Part model, mm, in its own coordinate system. A direction names the side the tool comes from. Give positions to 0.01 mm unless a question says otherwise; leave off trailing zeros. Order: outer loops, then holes, each group sorted by start corner. A loop starts at its lowest first (then second) coordinate and runs counter-clockwise, first axis right, second up. Notation, with made-up numbers: M 56,0.5 L 68,0.5 A22 ccw 68,24.5 Z; hole C -21,78.25 d4. An arc over 180 degrees is marked long. Return JSON: item names as keys, results as strings.
Autodesk Inventor part; units mm, degrees
ref_plane "YZ Plane" through (0, 0, 0) normal (1, 0, 0) x (0, 1, 0)
ref_plane "XZ Plane" through (0, 0, 0) normal (0, 1, 0) x (-1, 0, 0)
ref_plane "XY Plane" through (0, 0, 0) normal (0, 0, 1) x (1, 0, 0)
sketch "Sketch1" plane through (0, 0, 0) normal (0, 1, 0) x (-1, 0, 0)
  line L0 (-20, -20) -> (20, -20)
  line L1 (20, -20) -> (20, 20)
  line L2 (20, 20) -> (-20, 20)
  line L3 (-20, 20) -> (-20, -20)
  line L4 (-20, -20) -> (20, 20) construction
  line L5 (20, -20) -> (-20, 20) construction
  point P0 (0, 0)
  dimension "d2" = 40
  dimension "d3" = 40
extrude "Extrusion1" add sketch "Sketch1" along normal blind 5
sketch "Sketch2" plane through (0, 5, 0) normal (0, 1, 0) x (1, 0, 0)
  line L0 (-20, 20) -> (-20, -20)
  line L1 (-20, -20) -> (20, -20)
  line L2 (20, -20) -> (20, 20)
  line L3 (20, 20) -> (-20, 20)
  line L4 (17, 17) -> (-17, 17)
  line L5 (-17, 17) -> (-17, -17)
  line L6 (-17, -17) -> (17, -17)
  line L7 (17, -17) -> (17, 17)
  line L8 (17, 17) -> (-17, -17) construction
  line L9 (-17, 17) -> (17, -17) construction
  line L10 (15, 15) -> (-15, 15)
  line L11 (-15, 15) -> (-15, -15)
  line L12 (-15, -15) -> (15, -15)
  line L13 (15, -15) -> (15, 15)
  line L14 (15, 15) -> (-15, -15) construction
  line L15 (-15, 15) -> (15, -15) construction
  point P0 (0, 0)
  dimension "d6" = 3
  dimension "d7" = 2
  dimension "d52" = 3
  dimension "d53" = 2
extrude "Extrusion2" add sketch "Sketch2" along normal blind 40 contours L7 L6 L5 L4
fillet "Fillet1" radius 1 1 edges at (20, 2.5, 20)
fillet "Fillet2" radius 1 1 edges at (20, 2.5, -20)
fillet "Fillet3" radius 1 1 edges at (-20, 2.5, 20)
fillet "Fillet4" radius 1 1 edges at (-20, 2.5, -20)
fillet "Fillet5" radius 1 1 edges at (-17, 25, 17)
fillet "Fillet6" radius 1 1 edges at (17, 25, 17)
fillet "Fillet7" radius 1 1 edges at (17, 25, -17)
fillet "Fillet8" radius 1 1 edges at (-17, 25, -17)
sketch "Sketch3" plane through (0, 45, 0) normal (0, 1, 0) x (1, 0, 0)
  arc A0 (-16, 17) -> (-17, 16) centre (-16, 16) ccw
  line L0 (-17, 16) -> (-17, -16)
  arc A1 (-17, -16) -> (-16, -17) centre (-16, -16) ccw
  line L1 (-16, -17) -> (16, -17)
  arc A2 (16, -17) -> (17, -16) centre (16, -16) ccw
  line L2 (17, -16) -> (17, 16)
  arc A3 (17, 16) -> (16, 17) centre (16, 16) ccw
  line L3 (16, 17) -> (-16, 17)
  line L4 (15, 15) -> (15, -15)
  line L5 (15, -15) -> (-15, -15)
  line L6 (-15, -15) -> (-15, 15)
  line L7 (-15, 15) -> (15, 15)
  line L8 (-16.5, -10) -> (-15.5, -10)
  line L9 (-15.5, -10) -> (-15.5, 10)
  line L10 (-15.5, 10) -> (-16.5, 10)
  line L11 (-16.5, 10) -> (-16.5, -10)
  line L12 (-16.5, 10) -> (-15.5, 10)
  line L13 (-15.5, 10) -> (-15.5, -10)
  line L14 (-15.5, -10) -> (-16.5, -10)
  line L15 (-16.5, -10) -> (-16.5, 10)
  line L16 (-10, 16.5) -> (10, 16.5)
  line L17 (10, 16.5) -> (10, 15.5)
  line L18 (10, 15.5) -> (-10, 15.5)
  line L19 (-10, 15.5) -> (-10, 16.5)
  line L20 (10, 16.5) -> (-10, 16.5)
  line L21 (-10, 16.5) -> (-10, 15.5)
  line L22 (-10, 15.5) -> (10, 15.5)
  line L23 (10, 15.5) -> (10, 16.5)
  line L24 (15.5, 10) -> (16.5, 10)
  line L25 (16.5, 10) -> (16.5, -10)
  line L26 (16.5, -10) -> (15.5, -10)
  line L27 (15.5, -10) -> (15.5, 10)
  line L28 (15.5, -10) -> (16.5, -10)
  line L29 (16.5, -10) -> (16.5, 10)
  line L30 (16.5, 10) -> (15.5, 10)
  line L31 (15.5, 10) -> (15.5, -10)
  line L32 (10, -15.5) -> (-10, -15.5)
  line L33 (-10, -15.5) -> (-10, -16.5)
  line L34 (-10, -16.5) -> (10, -16.5)
  line L35 (10, -16.5) -> (10, -15.5)
  line L36 (-10, -15.5) -> (10, -15.5)
  line L37 (10, -15.5) -> (10, -16.5)
  line L38 (10, -16.5) -> (-10, -16.5)
  line L39 (-10, -16.5) -> (-10, -15.5)
  point P0 (0, 0)
  point P1 (-16, 10)
  point P2 (-16, -10)
  point P3 (16, 10)
  dimension "d18" = 1
  dimension "d19" = 20
  dimension "d20" = 0.5
  dimension "d21" = 7
  dimension "d22" = 7
  dimension "d23" = 0.5
  dimension "d24" = 1
  dimension "d25" = 20
  dimension "d26" = 20
  dimension "d27" = 1
  dimension "d28" = 0.5
  dimension "d29" = 7
  dimension "d30" = 20
  dimension "d31" = 1
  dimension "d32" = 0.5
  dimension "d33" = 7
  dimension "d34" = 1
  dimension "d35" = 20
  dimension "d36" = 0.5
  dimension "d37" = 7
  dimension "d38" = 1
  dimension "d39" = 20
  dimension "d40" = 7
  dimension "d41" = 0.5
  dimension "d42" = 20
  dimension "d43" = 1
  dimension "d44" = 0.5
  dimension "d45" = 7
  dimension "d46" = 20
  dimension "d47" = 1
  dimension "d48" = 0.5
  dimension "d49" = 7
extrude "Extrusion3" cut sketch "Sketch3" against normal blind 1 contours L11 L10 L9 L8 | L16 L17 L18 L19 | L24 L25 L26 L27 | L35 L34 L33 L32
properties part number "block_main" material "PC/ABS Plastic"
Q1. Pin check, flat tips, straight feed: pin 1 (6 mm diameter, centred on x = 16, y = 13, fed in from +Z); pin 2 (15 mm diameter, centred on x = 0, y = 27, fed in from -Z); pin 3 (6 mm diameter, centred on y = 21.5, z = -1, fed in from -X). Stop position of each tip, or through.
Established:
{"pin 1": "stops at z = 17", "pin 2": "stops at z = -17", "pin 3": "stops at x = -17"}
Q2. Band-saw the part on B-B (y = 16). Give the cut face in (x, z).
Established:
{"outline": "M -17,-16 A1 ccw -16,-17 L 16,-17 A1 ccw 17,-16 L 17,16 A1 ccw 16,17 L -16,17 A1 ccw -17,16 Z; hole M -15,-15 L 15,-15 L 15,15 L -15,15 Z"}
Q3. Band-saw the part on A-A (z = 12). Give the cut face in (x, y), then the cut area to 3 significant figures.
Established:
{"outline": "M -20,0 L 20,0 L 20,5 L 17,5 L 17,45 L 15,45 L 15,5 L -15,5 L -15,45 L -17,45 L -17,5 L -20,5 Z", "area": "360 mm²"}
Q4. Band-saw the part on C-C (x = 3). Give the cut face in (y, z), then the cut area to 3 significant figures.
Established:
{"outline": "M 0,-20 L 5,-20 L 5,-17 L 45,-17 L 45,-16.5 L 44,-16.5 L 44,-15.5 L 45,-15.5 L 45,-15 L 5,-15 L 5,15 L 45,15 L 45,15.5 L 44,15.5 L 44,16.5 L 45,16.5 L 45,17 L 5,17 L 5,20 L 0,20 Z", "area": "358 mm²"}
Q5. Two-plate mould, pull along Z, no slides. Class faces 5 (the flat face through (-15.2, 45, -0.1)), 6 (the flat face through (0, 25, 17)), 7 (the flat face through (0, 5, 0)): +Z half, -Z half, draft (parallel to the pull), parting line (faces both ways), or undercut.
Established:
{"face 5": "draft", "face 6": "+Z half", "face 7": "undercut"}
Q6. 3-axis set-ups, long thin cutter, end or side, ignore diameter. For faces 1 (the flat face through (0, 25, -15)), 2 (the flat face through (0, 25, -17)), 3 (the flat face through (-17, 25, 0)), 4 (the flat face through (17, 25, 0)): which of +Z, -Z, +X, -X, +Y, -Y reach the whole face in a straight line?
Established:
{"face 1": "+Y", "face 2": "-Z, +X, -X, +Y", "face 3": "+Z, -Z, -X, +Y", "face 4": "+Z, -Z, +X, +Y"}
Q7. Probe line 1 along Z through (x, y) = (11.5, 13); line 2 along Y through (x, z) = (17.5, -10.5). List the from-to ranges inside material, lowest first.
Established:
{"line 1": "z = -17 to -15, 15 to 17", "line 2": "y = 0 to 5"}
Q8. Band-saw the part on D-D (z = -1). Give the cut face in (x, y).
Established:
{"outline": "M -20,0 L 20,0 L 20,5 L 17,5 L 17,45 L 16.5,45 L 16.5,44 L 15.5,44 L 15.5,45 L 15,45 L 15,5 L -15,5 L -15,45 L -15.5,45 L -15.5,44 L -16.5,44 L -16.5,45 L -17,45 L -17,5 L -20,5 Z"}
